Source: CAD feature listing. Evaluate the final solid. Frame: model axes, mm. Face numbers are marked on the shaded views. A direction names the side the tool comes from. Round coordinates to 2 decimals unless told otherwise and drop trailing zeros. Order: outer loops, then holes, each group sorted by start corner. A loop starts at its lowest first (then second) coordinate and runs counter-clockwise, first axis right, second up. Notation, with made-up numbers: (46.5, 87) - (75.5, 87) arc R4 cw to (75.5, 93) - close; hole circle Ø6 at (64.5, 16.25). An arc over 180 degrees is marked (long way). Return JSON: item names as keys, results as strings. Group by question number.
1) Section A-A, the plane x = 0. Return loops of the section in (y, z) (1 decimal).
2) Contact query for flat-ended pins moving along their axis: P1, Ø1.5, axis at x = -0.5, y = 4, coming from the -Z side; P2, Ø6.5, axis at x = 0, z = -5.5, coming from the +Y side; P3, Ø2, axis at x = -2, z = -11, coming from the -Y side. Output: stop coordinate, or through.
3) Section C-C, the plane z = -4.5. Return loops of the section in (x, y).
4) Mould query, pull axis X, two halves, no side actions, for the marked faces 1, 2 and 3. Classes: pulls with the +X half, pulls with the -X half, needs draft (parallel to the pull), parting line crosses it, or undercut.
5) Ray query, line 1 (X direction, y = -0.75, z = -0.5); line 2 (Y direction, x = 1, z = -1.75); line 3 (Z direction, x = 5.25, y = 9.75). Return the intervals inside material, ascending. Write a range as from..to.
6) Section B-B, the plane y = 9.5. Return loops of the section in (x, z), plus the area to 3 significant figures.
7) Access query for the marked faces 4, 5 and 6. Directions: +Z, -Z, +X, -X, +Y, -Y. A direction counts if a zero-diameter tool reaches every point of the face in a straight line with its end or side. Return the directions, or none.
8) Section D-D, the plane x = -3. Return loops of the section in (y, z) (3 decimals), plus the area to 3 significant figures.
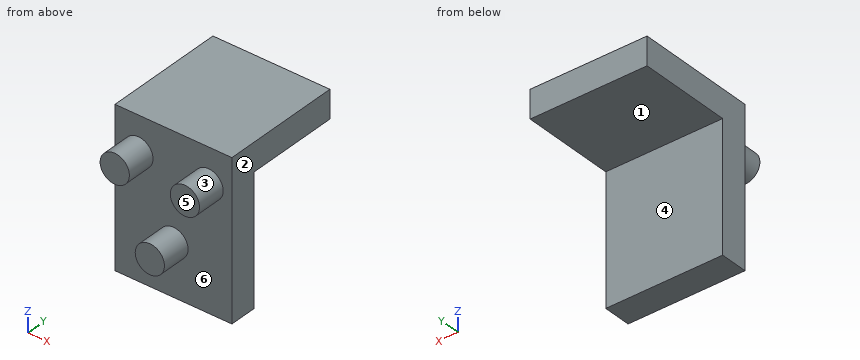
```python
from build123d import *

# Parameters (mm, degrees)
SKETCH2_W           = 12.7
SKETCH2_H           = 6.858
BOSS_EXTRUDE1_DEPTH = 3
SKETCH3_R           = 1.5875
BOSS_EXTRUDE2_DEPTH = 3.175
SKETCH4_W           = 12.7
SKETCH4_H           = 3.81
BOSS_EXTRUDE3_DEPTH = 10.16
SKETCH8_W           = 12.7
SKETCH8_H           = 3
BOSS_EXTRUDE6_DEPTH = 10.16
SKETCH11_R          = 1.5875
BOSS_EXTRUDE7_DEPTH = 3.175
SKETCH12_W          = 12.7
SKETCH12_H          = 0.762
CUT_EXTRUDE1_DEPTH  = 10.16


with BuildPart() as part:
    # Sketch2 → Boss-Extrude1 (new body)
    with BuildSketch(Plane(origin=(0, 0, 0), x_dir=(1, 0, 0), z_dir=(0, 1, 0))):
        Rectangle(SKETCH2_W, SKETCH2_H)
    extrude(amount=BOSS_EXTRUDE1_DEPTH)

    # Sketch3 → Boss-Extrude2 (add)
    with BuildSketch(Plane.XZ):
        with Locations(Location((3.81, -0.381, 0), (0, 0, 90))):
            Circle(SKETCH3_R)
        with Locations(Location((-3.81, -0.381, 0), (0, 0, 90))):
            Circle(SKETCH3_R)
    extrude(amount=BOSS_EXTRUDE2_DEPTH)

    # Sketch4 → Boss-Extrude3 (add)
    with BuildSketch(Plane(origin=(0, 3, 0), x_dir=(1, 0, 0), z_dir=(0, 1, 0))):
        with Locations((0, -1.524)):
            Rectangle(SKETCH4_W, SKETCH4_H)
    extrude(amount=BOSS_EXTRUDE3_DEPTH)

    # Sketch8 → Boss-Extrude6 (add)
    with BuildSketch(Plane(origin=(0, 0, -3.429), x_dir=(-1, 0, 0), z_dir=(0, 0, -1))):
        with Locations((0, 1.5)):
            Rectangle(SKETCH8_W, SKETCH8_H)
    extrude(amount=BOSS_EXTRUDE6_DEPTH)

    # Sketch11 → Boss-Extrude7 (add)
    with BuildSketch(Plane.XZ):
        with Locations(Location((0, -8.001, 0), (0, 0, 90))):
            Circle(SKETCH11_R)
    extrude(amount=BOSS_EXTRUDE7_DEPTH)

    # Sketch12 → Cut-Extrude1 (cut)
    with BuildSketch(Plane(origin=(0, 13.16, 0), x_dir=(1, 0, 0), z_dir=(0, 1, 0))):
        Rectangle(SKETCH12_W, SKETCH12_H)
    extrude(amount=-CUT_EXTRUDE1_DEPTH, mode=Mode.SUBTRACT)


solid = part.part
```
Geometry check:
{
 "1": {"outline": "(-3.2, -9.6) - (0, -9.6) - (0, -13.6) - (3, -13.6) - (3, 0.4) - (13.2, 0.4) - (13.2, 3.4) - (0, 3.4) - (0, -6.4) - (-3.2, -6.4) - close"},
 "2": {"P1": "z = 0.38", "P2": "y = 3", "P3": "y = 0"},
 "3": {"outline": "(-6.35, 0) - (6.35, 0) - (6.35, 3) - (-6.35, 3) - close"},
 "4": {"face 1": "needs draft", "face 2": "pulls with the +X half", "face 3": "undercut"},
 "5": {"line 1": "-5.39..-2.23, 2.23..5.39", "line 2": "0..3", "line 3": "0.38..3.43"},
 "6": {"outline": "(-6.35, 0.38) - (6.35, 0.38) - (6.35, 3.43) - (-6.35, 3.43) - close", "area": "38.7 mm2"},
 "7": {"face 4": "-Z, +X, -X, +Y", "face 5": "+Z, -Z, +X, -X, -Y", "face 6": "-Y"},
 "8": {"outline": "(-3.175, -1.746) - (0, -1.746) - (0, -13.589) - (3, -13.589) - (3, 0.381) - (13.16, 0.381) - (13.16, 3.429) - (0, 3.429) - (0, 0.984) - (-3.175, 0.984) - close", "area": "90.7 mm2"}
}
